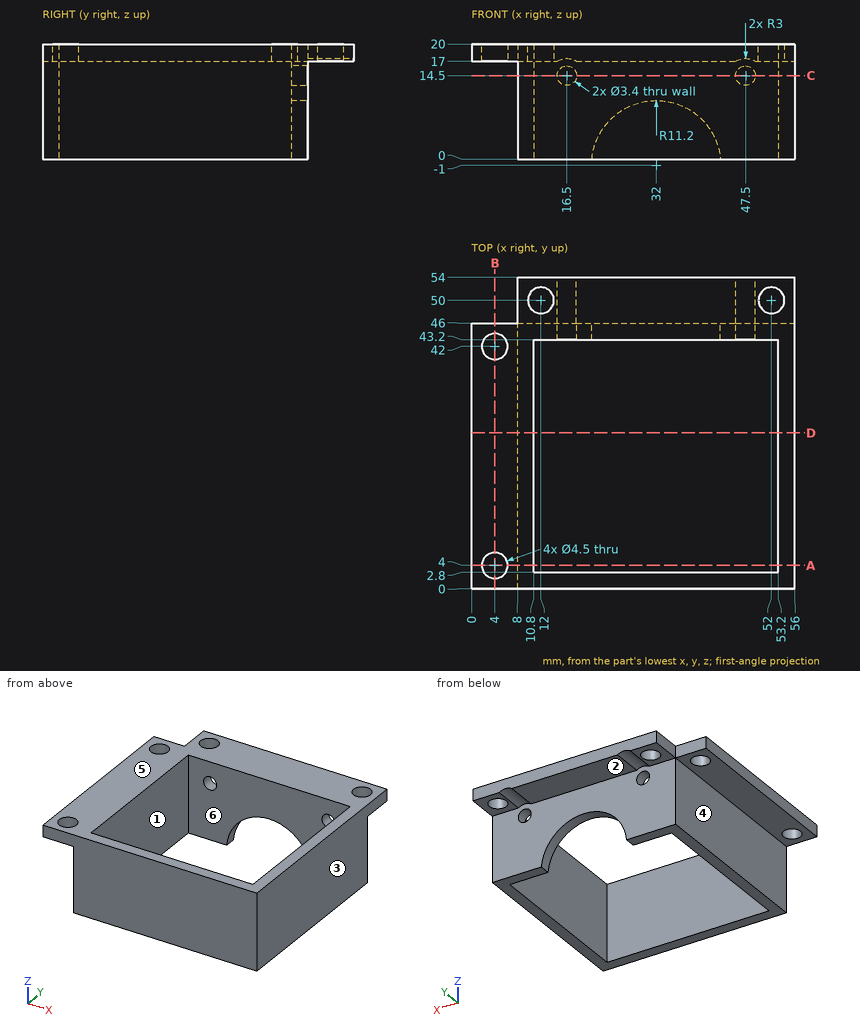
Drawing for the job (mm, zero at the part's lowest x, y, z). A direction names the side the tool comes from. Round coordinates to 2 decimals unless told otherwise and drop trailing zeros. Write each loop counter-clockwise with the first axis right and the second up, starting at its lowest first coordinate (ties: lowest second). Pieces come first, ordered by that corner, then holes. Notation, with made-up numbers: M -39.75,22 L -14.75,22 A9 cw -14.75,38 Z; hole C 43.5,43 d2. An arc over 180 degrees is marked long. Answer as a JSON object with one key per item and string values. Group by question number.
(1) Mould opens along X. For the marked faces 1, 2 and 3 say: pulls with the +X half, pulls with the -X half, needs draft (parallel to the pull), parting line crosses it, or undercut.
(2) Cut at C-C (z = 14.5). Give the cut face in (x, y), and give its area (3 significant figures).
(3) Cut at D-D (y = 27). Give the cut face in (x, z), and give its area (3 significant figures).
(4) Cut at A-A (y = 4). Give the cut face in (x, z), and give its area (4 significant figures).
(5) Cut at B-B (x = 4). Give the cut face in (y, z).
(6) Which spindle directions (+Z, -Z, +X, -X, +Y, -Y) get a long thin tool onto all of the face, cutting with end or side? Do the marked faces 4, 5 and 6. Say none if no direction does.
(7) Flat gauge pins, fed straight in: pin 1 (5.5 mm diameter, centred on x = 53.5, y = 49.5, fed in from -Z); pin 2 (4.5 mm diameter, centred on x = 47.5, z = 14.5, fed in from -Y); pin 3 (6 mm diameter, centred on x = 35.5, z = 5, fed in from +Y); pin 4 (6 mm diameter, centred on y = 41, z = 3.5, fed in from -X). Where does each tip first touch, or does it go through?
(8) Drill centre lines: L1, parallel to Y at x = 4, z = 17.6; L2, parallel to Y at x = 12, z = 18.05; L3, parallel to Y at x = 41, z = 17.25. Where is each one in solid material? Low to high.
Responses:
{
 "1": {"face 1": "undercut", "face 2": "needs draft", "face 3": "pulls with the +X half"},
 "2": {"outline": "M 8,0 L 56,0 L 56,46 L 49.2,46 L 49.2,43.2 L 53.2,43.2 L 53.2,2.8 L 10.8,2.8 L 10.8,43.2 L 14.8,43.2 L 14.8,46 L 8,46 Z; M 18.2,43.2 L 45.8,43.2 L 45.8,46 L 18.2,46 Z", "area": "476 mm2"},
 "3": {"outline": "M 0,17 L 8,17 L 8,0 L 10.8,0 L 10.8,20 L 0,20 Z; M 53.2,0 L 56,0 L 56,20 L 53.2,20 Z", "area": "136 mm2"},
 "4": {"outline": "M 0,17 L 1.75,17 L 1.75,20 L 0,20 Z; M 6.25,17 L 8,17 L 8,0 L 10.8,0 L 10.8,20 L 6.25,20 Z; M 53.2,0 L 56,0 L 56,20 L 53.2,20 Z", "area": "122.5 mm2"},
 "5": {"outline": "M 0,17 L 1.75,17 L 1.75,20 L 0,20 Z; M 6.25,17 L 39.75,17 L 39.75,20 L 6.25,20 Z; M 44.25,17 L 46,17 L 46,20 L 44.25,20 Z"},
 "6": {"face 4": "-Z, -X, +Y, -Y", "face 5": "+Z, +X, -X, +Y, -Y", "face 6": "+Z, -Z"},
 "7": {"pin 1": "stops at z = 17", "pin 2": "stops at y = 0", "pin 3": "stops at y = 2.8", "pin 4": "stops at x = 8"},
 "8": {"L1": "y = 0 to 1.75, 6.25 to 39.75, 44.25 to 46", "L2": "y = 0 to 2.8, 43.2 to 47.75, 52.25 to 54", "L3": "y = 0 to 2.8, 43.2 to 54"}
}
